from build123d import *

# Parameters (mm, degrees)
SKETCH_1_W      = 14.3
SKETCH_1_H      = 15.3
EXTRUDE_1_DEPTH = 0.5
SKETCH_2_W      = 4.2
SKETCH_2_H      = 7.5
SKETCH_2_W_2    = 4.7
EXTRUDE_2_DEPTH = 0.5
FILLET_1_R      = 1.5
FILLET_2_R      = 0.5
SKETCH_3_W      = 12
SKETCH_3_H      = 12
EXTRUDE_3_DEPTH = 4
FILLET_3_R      = 1
SKETCH_4_R      = 1
EXTRUDE_4_DEPTH = 0.1
FILLET_4_R      = 0.5


with BuildPart() as part:
    # ｽｹｯﾁ1 → ﾎﾞｽ - 押し出し1 (new body)
    with BuildSketch(Plane.XY):
        Rectangle(SKETCH_1_W, SKETCH_1_H)
    extrude(amount=EXTRUDE_1_DEPTH)

    # ｽｹｯﾁ2 → ﾎﾞｽ - 押し出し2 (add)
    with BuildSketch(Plane.XY.offset(0.5)):
        with Locations((-9.25, -1.1)):
            Rectangle(SKETCH_2_W, SKETCH_2_H)
        with Locations((9.5, -1.1)):
            Rectangle(SKETCH_2_W_2, SKETCH_2_H)
    extrude(amount=-EXTRUDE_2_DEPTH)

    # ﾌｨﾚｯﾄ1
    fillet_1_edges = [part.edges().sort_by_distance(p)[0] for p in [
        (-7.15, 2.65, 0.25),
        (-7.15, -4.85, 0.25),
        (-11.35, -4.85, 0.25),
        (-11.35, 2.65, 0.25),
        (7.15, -4.85, 0.25),
        (7.15, 2.65, 0.25),
        (11.85, 2.65, 0.25),
        (11.85, -4.85, 0.25),
        (7.15, 7.65, 0.25),
    ]]
    fillet(fillet_1_edges, radius=FILLET_1_R)

    # ﾌｨﾚｯﾄ2
    fillet_2_edges = [part.edges().sort_by_distance(p)[0] for p in [
        (-7.15, 7.65, 0.25),
    ]]
    fillet(fillet_2_edges, radius=FILLET_2_R)

    # ｽｹｯﾁ3 → ﾎﾞｽ - 押し出し3 (add)
    with BuildSketch(Plane.XY.offset(0.5)):
        with Locations((0.05, 0.35)):
            Rectangle(SKETCH_3_W, SKETCH_3_H)
    extrude(amount=EXTRUDE_3_DEPTH)

    # ﾌｨﾚｯﾄ3
    fillet_3_edges = [part.edges().sort_by_distance(p)[0] for p in [
        (-5.95, 6.35, 2.5),
        (-5.95, -5.65, 2.5),
        (6.05, -5.65, 2.5),
        (6.05, 6.35, 2.5),
    ]]
    fillet(fillet_3_edges, radius=FILLET_3_R)

    # ｽｹｯﾁ4 → ﾎﾞｽ - 押し出し4 (add)
    with BuildSketch(Plane.XY.offset(4.5)):
        with Locations((0, -0.5)):
            Circle(SKETCH_4_R)
    extrude(amount=EXTRUDE_4_DEPTH)

    # ﾌｨﾚｯﾄ4
    # the kernel refuses this fillet: 0.5 mm, written as the material it takes off along each edge
    with BuildSketch(Plane(origin=(0, -0.5, 4.6), x_dir=(1, 0, 0), z_dir=(0, -1, 0))) as fillet_4_piece_1:
        with BuildLine():
            CenterArc((0.7, -0.5), FILLET_4_R, 53.130102354, 36.869897646)
            Line((0.7, 0), (0.7, 0.01))
            Line((0.7, 0.01), (1, 0.01))
            Line((1, 0.01), (1.01, 0))
            ThreePointArc((1.01, 0), (1.01, -0.05), (1.006, -0.092))
            Line((1.006, -0.092), (1, -0.1))
        make_face()
    revolve(axis=Axis((0, -0.5, 4.6), (0, 0, 1)), mode=Mode.SUBTRACT)


solid = part.part
Can you work these out from the model? Positions are in its coordinate system, mm. A direction names the side the tool comes from. Round coordinates to 2 decimals unless told otherwise and drop trailing zeros. Write each loop counter-clockwise with the first axis right and the second up, starting at its lowest first coordinate (ties: lowest second). Pieces come first, ordered by that corner, then holes. Notation, with made-up numbers: (33, 39) -> (56, 39) arc R16 ccw to (56, 63) -> close; hole circle Ø3 at (44, -34.5). An arc over 180 degrees is marked (long way). One line per question, with ' | ' between items. Start each with the question number.
1) If we mould it in two halves opening along X, with no side actions, what happens to faces 5 (the flat face through (6.05, 0, 2)), 6 (the cylindrical face through (-7.58, 3.1, 0.25)), 7 (the flat face through (0, 6.35, 2))? For each: released by +X, released by -X, zero draft, split by the parting line, or undercut.
2) Suppose I cut it at A-A on z = 2.75. Write out the boundary of the cut face in (x, y).
3) On a 3-axis mill with a long thin cutter (end or side, diameter ignored), from which of +Z, -Z, +X, -X, +Y, -Y can I reach the whole of each face in a straight line? I mean faces 1 (the cylindrical face through (-5.649, 6.065, 2.528)), 2 (the cylindrical face through (5.765, 6.049, 2.528)), 3 (the cylindrical face through (-5.649, -5.365, 2.528)), 4 (the flat face through (0, -5.65, 2)). Say none if no direction works.
4) I need wall thicknesses on line 1 (X direction, y = -4, z = 2.4); line 2 (Z direction, x = 0.5, y = -3); line 3 (Z direction, x = -8.5, y = 1). Which ranges of each line are inside material? Lowest first, please. Write a range as [from, to].
5) Suppose I cut it at C-C on x = -7.75. Write out the boundary of the cut face in (y, z), then the cut area to 3 significant figures.
6) I'm going to push flat-ended pins straight in: P1, Ø0.6, axis at x = -9, z = 0, coming from the +Y side; P2, Ø6, axis at x = 9, y = 3, coming from the -Z side; P3, Ø1, axis at x = 4, z = 2.5, coming from the +Y side; P4, Ø7.5, axis at x = -4.5, y = -0.5, coming from the +Z side. Where does each tip first touch, or does it pass through?
7) Suppose I cut it at B-B on y = 4.75. Write out the boundary of the cut face in (x, z), then the cut area to 4 significant figures.
8) Suppose I cut it at D-D on x = 10. Write out the boundary of the cut face in (y, z).
Return value:
1) face 5: released by +X | face 6: released by -X | face 7: zero draft
2) outline: (-5.95, -4.65) arc R1 ccw to (-4.95, -5.65) -> (5.05, -5.65) arc R1 ccw to (6.05, -4.65) -> (6.05, 5.35) arc R1 ccw to (5.05, 6.35) -> (-4.95, 6.35) arc R1 ccw to (-5.95, 5.35) -> close
3) face 1: +Z, -X, +Y | face 2: +Z, +X, +Y | face 3: +Z, -X, -Y | face 4: +Z, +X, -X, -Y
4) line 1: x = [-5.95, 6.05] | line 2: z = [0, 4.5] | line 3: z = [0, 0.5]
5) outline: (-5.15, 0) -> (2.95, 0) -> (2.95, 0.5) -> (-5.15, 0.5) -> close | area: 4.05 mm2
6) P1: stops at y = 2.65 | P2: stops at z = 0 | P3: stops at y = 6.35 | P4: stops at z = 4.6
7) outline: (-7.15, 0) -> (7.15, 0) -> (7.15, 0.5) -> (6.05, 0.5) -> (6.05, 4.5) -> (-5.95, 4.5) -> (-5.95, 0.5) -> (-7.15, 0.5) -> close | area: 55.15 mm2
8) outline: (-4.85, 0) -> (2.65, 0) -> (2.65, 0.5) -> (-4.85, 0.5) -> close
